Part print with two shaded views. Sizes in mm from the minimum x, y, z corner. A direction names the side the tool comes from. Give positions to 0.01 mm unless a question says otherwise; leave off trailing zeros.
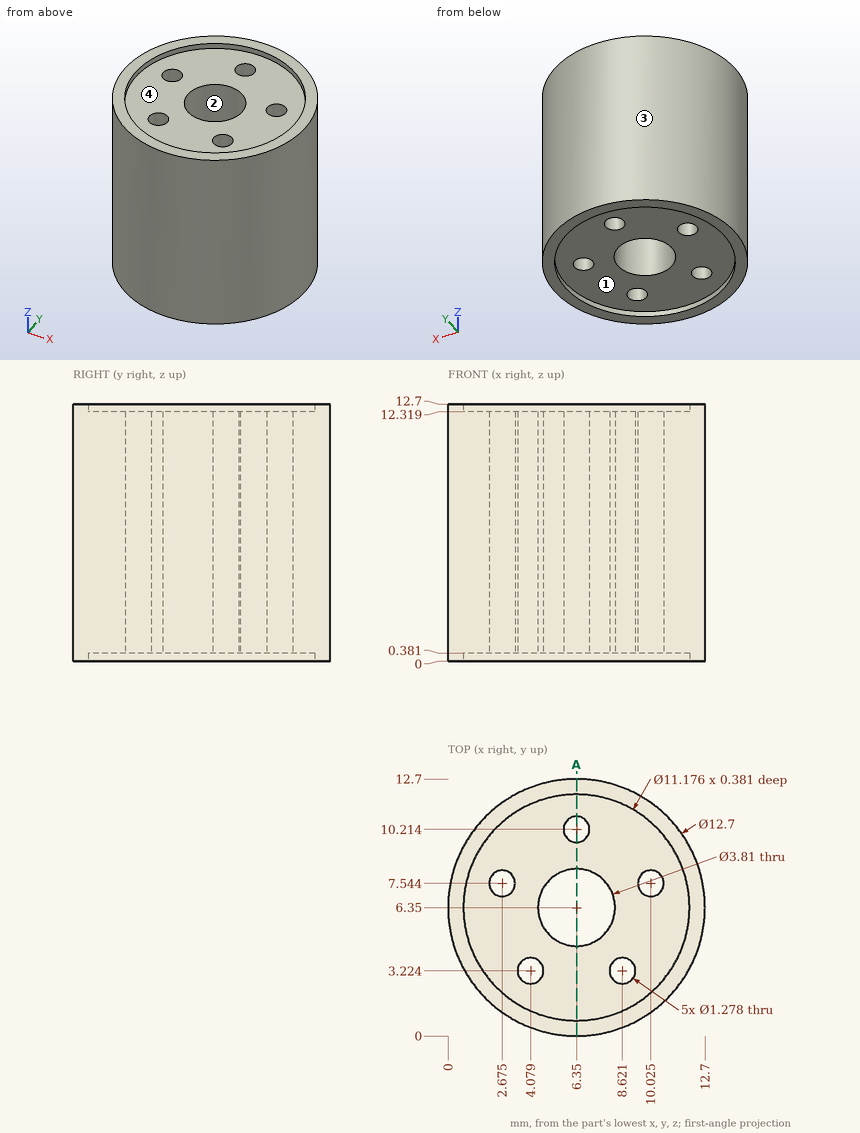
1) Drill centre lines: L1, parallel to Y at x = 6.35, z = 7.5 (1 decimal); L2, parallel to Y at x = 6.35, z = 0.2; L3, parallel to Y at x = 6.75, z = 6.25 (1 decimal). Where is each one in solid material? Low to high.
Check result:
L1: y = 0 to 4.4, 8.3 to 9.6, 10.9 to 12.7
L2: y = 0 to 0.76, 11.94 to 12.7
L3: y = 0 to 4.5, 8.2 to 9.7, 10.7 to 12.7
2) Mould opens along Y. For the marked faces 3 and 4 say: +Y half, -Y half, draft (parallel to the pull), parting line (faces both ways), or undercut.
Check result:
face 3: parting line
face 4: undercut
3) 3-axis set-ups, long thin cutter, end or side, ignore diameter. For the marked faces 1 and 2: which of +Z, -Z, +X, -X, +Y, -Y reach the whole face in a straight line?
Check result:
face 1: -Z
face 2: +Z, -Z
4) Flat gauge pins, fed straight in: P1, Ø3.5, axis at x = 6.35, y = 6.35, coming from the +Z side; P2, Ø6, axis at x = 7, y = 6.5, coming from the -Z side; P3, Ø6, axis at y = 9.5, z = 10, coming from the -X side; P4, Ø1, axis at y = 9.5, z = 7, coming from the -X side. Where does each tip first touch, or does it go through?
Check result:
P1: passes through
P2: stops at z = 0.38
P3: stops at x = 0
P4: stops at x = 0.58
5) Saw through at A-A (x = 6.35). State how many separate pieces and enclosed holes the cut face has.
Check result:
separate pieces: 3
enclosed holes: 0
